from build123d import *

# Parameters (mm, degrees)
F1_DEPTH = 609.6


with BuildPart() as f1:
    # F0 (on Front) → F1 (new body, symmetric)
    with BuildSketch(Plane.XZ):
        with BuildLine():
            Line((0, 9.525), (0, 12.7))
            Line((0, 12.7), (-6.35, 12.7))
            Line((-6.35, 12.7), (-152.4, 0.762))
            Line((-152.4, 0.762), (-152.4, 0))
            Line((-152.4, 0), (-4.7625, 0))
            Line((-4.7625, 0), (-4.7625, 4.7625))
            ThreePointArc((-4.7625, 4.7625), (-3.367596, 8.130096), (0, 9.525))
        make_face()
        with BuildLine():
            Line((6.35, 12.7), (0, 12.7))
            Line((0, 12.7), (0, 9.525))
            ThreePointArc((0, 9.525), (3.367596, 8.130096), (4.7625, 4.7625))
            Line((4.7625, 4.7625), (4.7625, 0))
            Line((4.7625, 0), (152.4, 0))
            Line((152.4, 0), (152.4, 0.762))
            Line((152.4, 0.762), (6.35, 12.7))
        make_face()
    extrude(amount=F1_DEPTH, both=True)


solid = f1.part
Here's how the part is built. I have some questions about the finished solid (model axes, mm). Coordinates: 2 decimals unless noted, no trailing zeros. Write each loop counter-clockwise with the first axis right and the second up, starting at its lowest first coordinate (ties: lowest second). Pieces come first, ordered by that corner, then holes. Notation, with made-up numbers: (-34.5, 62.25) - (-13.5, 62.25) arc R20 cw to (-13.5, 69.25) - close; hole circle Ø1 at (15.25, 4.25). An arc over 180 degrees is marked (long way). Use one line per item in the form item = value.
1) I need wall thicknesses on line 1 (Z direction, x = 87, y = -116); line 2 (Z direction, x = -85.5, y = 116). Which ranges of each line are inside material? Lowest first, please.
Solved:
line_1 = 0 to 6.11
line_2 = 0 to 6.23
2) Suppose I cut it at B-B, the plane x = -131. Write out the boundary of the cut face in (y, z).
Solved:
outline = (-609.6, 0) - (609.6, 0) - (609.6, 2.51) - (-609.6, 2.51) - close
3) Suppose I cut it at C-C, the plane x = 121. Write out the boundary of the cut face in (y, z), plus the area to 3 significant figures.
Solved:
outline = (-609.6, 0) - (609.6, 0) - (609.6, 3.33) - (-609.6, 3.33) - close
area = 4,060 mm2
4) I'm going to push flat-ended pins straight in: P1, Ø3, axis at x = 79, y = 452.5, coming from the +Z side; P2, Ø4, axis at x = -118.5, z = 7.5, coming from the -Y side; P3, Ø2, axis at x = 89, y = 212.5, coming from the +Z side. Where does each tip first touch, or does it pass through?
Solved:
P1 = 6.88
P2 = through
P3 = 6.03
